Answer from the drawing. Dimensions are ordinates in mm from the lowest x, y and z of the part. A direction names the side the tool comes from. Give positions to 0.01 mm unless a question says otherwise; leave off trailing zeros. Write each loop counter-clockwise with the first axis right and the second up, starting at its lowest first coordinate (ties: lowest second). Pieces come first, ordered by that corner, then holes. Notation, with made-up numbers: M 51,88.5 L 64,88.5 A22 cw 64,123.5 Z; hole C 79.25,35 d1. An arc over 180 degrees is marked long. Answer as a JSON object with one key per item and string values.
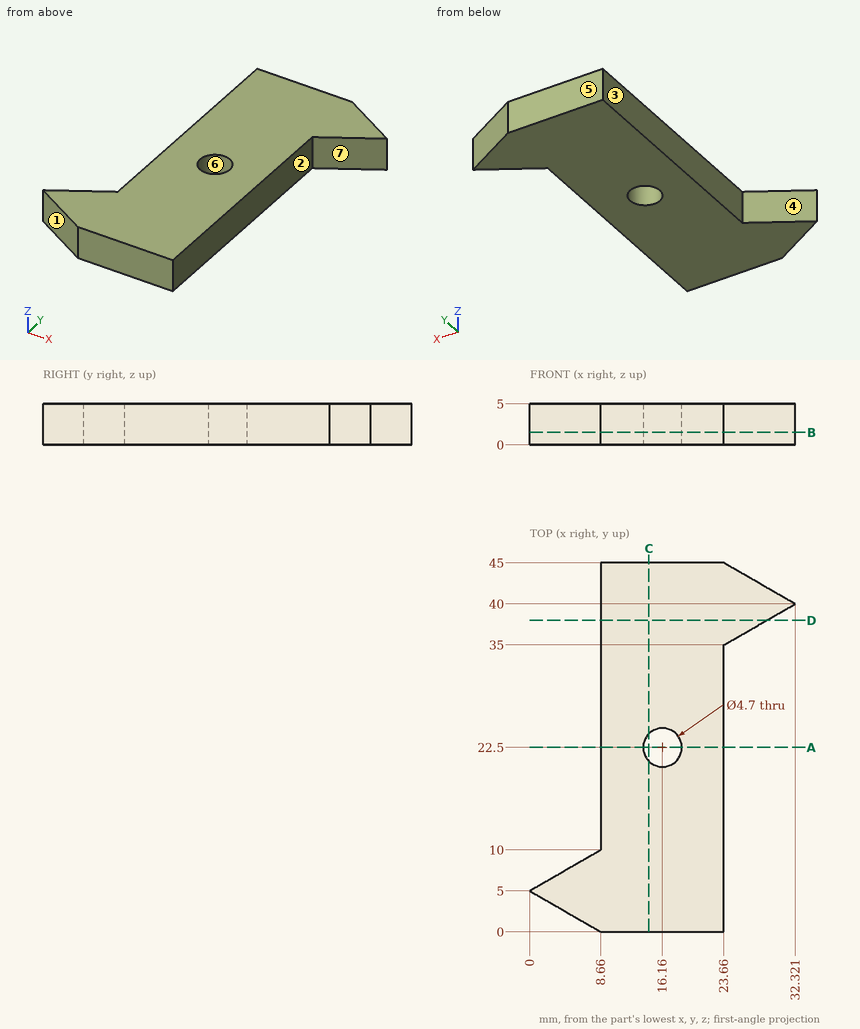
1. A cutting plane is placed at D-D, the plane y = 38. Give the vertices of the cut face in (x, z).
Verdict:
{"outline": "M 8.66,0 L 28.86,0 L 28.86,5 L 8.66,5 Z"}
2. A cutting plane is placed at A-A, the plane y = 22.5. Give the vertices of the cut face in (x, z), plus the area to 3 significant figures.
Verdict:
{"outline": "M 8.66,0 L 13.81,0 L 13.81,5 L 8.66,5 Z; M 18.51,0 L 23.66,0 L 23.66,5 L 18.51,5 Z", "area": "51.5 mm2"}
3. A cutting plane is placed at B-B, the plane z = 1.55. Give the vertices of the cut face in (x, y), plus the area to 3 significant figures.
Verdict:
{"outline": "M 0,5 L 8.66,0 L 23.66,0 L 23.66,35 L 32.32,40 L 23.66,45 L 8.66,45 L 8.66,10 Z; hole C 16.16,22.5 d4.7", "area": "744 mm2"}
4. Consider line 1 along X through (y, z) = (23, 4.85) (1 decimal); line 2 along X through (y, z) = (20, 3.45); line 3 along X through (y, z) = (24, 4.4). Determine where each line is inside the solid, lowest interval first.
Verdict:
{"line 1": "x = 8.7 to 13.9, 18.5 to 23.7", "line 2": "x = 8.66 to 23.66", "line 3": "x = 8.66 to 14.35, 17.97 to 23.66"}
5. A cutting plane is placed at C-C, the plane x = 14.5. Give the vertices of the cut face in (y, z), plus the area to 3 significant figures.
Verdict:
{"outline": "M 0,0 L 20.84,0 L 20.84,5 L 0,5 Z; M 24.16,0 L 45,0 L 45,5 L 24.16,5 Z", "area": "208 mm2"}
6. The mould has two halves that part along X. Classify the marked faces 4, 5, 6 and 7: released by +X, released by -X, zero draft, split by the parting line, or undercut.
Verdict:
{"face 4": "released by -X", "face 5": "zero draft", "face 6": "undercut", "face 7": "released by +X"}
7. Flat-ended cylindrical pins translate along their axes: pin 1 (1.5 mm diameter, centred on y = 32.5, z = 2, fed in from -X); pin 2 (2 mm diameter, centred on y = 32, z = 1, fed in from +X); pin 3 (4 mm diameter, centred on x = 16.16, y = 22.5, fed in from +Z). Find the tip coordinate at first contact, or state that the pin passes through.
Verdict:
{"pin 1": "stops at x = 8.66", "pin 2": "stops at x = 23.66", "pin 3": "passes through"}
8. For the marked faces 1, 2 and 3, determine the directions among +Z, -Z, +X, -X, +Y, -Y from which every point of the face is accessible in a straight line to the end or side of a thin tool.
Verdict:
{"face 1": "+Z, -Z, -X, -Y", "face 2": "+Z, -Z, +X, -Y", "face 3": "+Z, -Z, -X, +Y"}
